from build123d import *

# Parameters (mm, degrees)
SALIENTE_EXTRUIR2_DEPTH = 10
CROQUIS2_R              = 1.75
CORTAR_EXTRUIR1_DEPTH   = 3


with BuildPart() as part:
    # Croquis1 → Saliente-Extruir2 (new body)
    with BuildSketch(Plane.XY):
        with BuildLine():
            Line((5, -50), (-5, -50))
            Line((-5, -50), (-5, 46))
            ThreePointArc((-5, 46), (-3.828427125, 48.828427125), (-1, 50))
            Line((-1, 50), (1, 50))
            ThreePointArc((1, 50), (3.828427125, 48.828427125), (5, 46))
            Line((5, 46), (5, -50))
        make_face()
    extrude(amount=SALIENTE_EXTRUIR2_DEPTH)

    # Croquis2 → Cortar-Extruir1 (cut)
    with BuildSketch(Plane.XY.offset(10)):
        with Locations((0, 43.791816943)):
            Circle(CROQUIS2_R)
    extrude(amount=-CORTAR_EXTRUIR1_DEPTH, mode=Mode.SUBTRACT)


solid = part.part
Could you check a few things on this model? Use its own coordinates, in mm. A direction names the side the tool comes from. Round coordinates to 2 decimals unless told otherwise and drop trailing zeros. Use a Markdown table: item, result.
Q1. For faces 1 (the flat face through (0, -50, 5)), 2 (the cylindrical face through (-0.379, 42.083, 8.521)), which set-ups out of +Z, -Z, +X, -X, +Y, -Y let a thin tool reach every point of the face, with its end or its side?
Output values:
| item | result |
|---|---|
| face 1 | +Z, -Z, +X, -X, -Y |
| face 2 | +Z |
Q2. Please list where these lines run through material, in increasing order: L1, parallel to Y at x = 0, z = 7.95; L2, parallel to Y at x = 1.5, z = 8.25; L3, parallel to Y at x = 2.75, z = 8.25.
Output values:
| item | result |
|---|---|
| L1 | -50 to 42.04, 45.54 to 50 |
| L2 | -50 to 42.89, 44.69 to 49.97 |
| L3 | -50 to 49.6 |
Q3. For pin 1 (1 mm diameter, centred on x = 0, y = 44, fed in from +Z), with a flat end and sliding along its axis, tell me the tip position at first contact or that it passes through.
Output values:
| item | result |
|---|---|
| pin 1 | z = 7 |
Q4. Thinking about a two-plate mould opening in X: for faces 3 (the cylindrical face through (3.797, 48.859, 4.93)), 4 (the flat face through (0, 44, 7)), 5 (the flat face through (0, 1, 0)), 6 (the cylindrical face through (-3.859, 48.797, 4.93)), which applies, released by +X, released by -X, zero draft, split by the parting line, or undercut?
Output values:
| item | result |
|---|---|
| face 3 | released by +X |
| face 4 | undercut |
| face 5 | zero draft |
| face 6 | released by -X |
